Design review of the part built by this model. Coordinates are the model's own, in mm. A direction names the side the tool comes from. Coordinates: 2 decimals unless noted, no trailing zeros. Write each loop counter-clockwise with the first axis right and the second up, starting at its lowest first coordinate (ties: lowest second). Pieces come first, ordered by that corner, then holes.
Q1. The part is to be moulded in two halves that separate along X. For faces 1 (the face through (0, 4, 0)), 2 (the face through (-0.29, -2.23, 1.23)), 3 (the face through (2.64, -8.44, -0.99)), say which applies: +X half, -X half, draft (parallel to the pull), parting line (faces both ways), or undercut.
Q2. Add section B-B, the plane z = -1.6. Give the boundary of the cut face in (x, y) (3 decimals).
Q3. Add section D-D, the plane z = 1.5. Give the boundary of the cut face in (x, y), plus the area to 3 significant figures.
Q4. Add section C-C, the plane x = 4.25. Give the boundary of the cut face in (y, z), plus the area to 3 significant figures.
Q5. Clearance check with flat-ended pins moving along their axes: pin 1 Ø10 at (x, y) = (-2, 12) entering from +Z; pin 2 Ø2 at (x, z) = (-5, -1) entering from -Y; pin 3 Ø1 at (x, z) = (4.5, -1) entering from +Y. State where each tip first meets the part, or that it passes through.
Q6. Add section A-A, the plane y = 0. Give the boundary of the cut face in (x, z) (3 decimals).
Q7. To check wall thickness, follow probe 1 along X at (y, z) = (0, 1.75); probe 2 along Z at (x, y) = (-2, -6). State the ranges of each line that lie inside material, in increasing order.
Q8. Machinability: for faces 4 (the face through (-5, -2, -1)), 5 (the face through (0, 0, 0)), 6 (the face through (5, 2, -1)), 7 (the face through (5, -2, -1)), which of the approach directions +Z, -Z, +X, -X, +Y, -Y give a long, thin tool a straight path to every point of the face, cutting with its end or side? Answer none if there is none.
Autodesk Fusion 360 part; units mm, degrees
sketch "Sketch1" plane through (0, 0, 0) normal (0, 0, 1) x (1, 0, 0)
  circle A0 centre (0, 0) radius 3.5
  circle A1 centre (0, 0) radius 2.25
  circle A2 centre (0, 16.5) radius 2
  circle A3 centre (0, -14.5) radius 2
  circle A4 centre (-6.375, 0) radius 2
  circle A5 centre (6.375, 0) radius 2
  line L0 (0, 0) -> (0, 16.5) construction
  line L1 (-1.9917, 16.6818) -> (-3.4855, 0.3182)
  line L2 (-1.9893, -14.7069) -> (-3.4812, -0.3621)
  line L3 (1.9917, 16.6818) -> (3.4855, 0.3182)
  line L4 (1.9893, -14.7069) -> (3.4812, -0.3621)
  line L5 (-6.375, 2) -> (6.375, 2)
  line L6 (6.375, 2) -> (6.375, -2) construction
  line L7 (6.375, -2) -> (-6.375, -2)
  line L8 (-6.375, -2) -> (-6.375, 2) construction
  circle A6 centre (0, 0) radius 1.25
  circle A7 centre (0, 5) radius 0.625
  circle A8 centre (0, -5) radius 0.625
  point P0 (0, -16.5)
  point P1 (0, 18.5)
  point P2 (-8.375, 0)
  point P3 (8.375, 0)
  dimension "d1" = 7
  dimension "d2" = 4.5
  dimension "d5" = 35
  dimension "d7" = 4
  dimension "d8" = 16.75
  dimension "d9" = 14.5
  dimension "d12" = 2.5
  dimension "d14" = 5
  dimension "d15" = 1.25
  dimension "d22" = 5
extrude "Extrude1" add sketch "Sketch1" along normal blind 2.5 contours A0 A1 L5 L7 | A0 A1 L5 | A0 A1 L7 | A0 A1 L5 L7
extrude "Extrude2" add sketch "Sketch1" against normal blind 2 contours A0 A1 L5 L7 | A0 A5 L3 L4 L5 L7 | A0 L3 L5 | A0 L4 L7 | A0 A1 L5 | A0 A2 L1 L3 L5 | A0 A3 L2 L4 L7 | A0 A1 L7 | A0 A1 L5 L7 | A0 L1 L5 | A1 L5 | A1 L5 L7 | A2 | A5 | A0 L2 L7 | A1 L7 | A3 | A0 A4 L1 L2 L5 L7 | A4 | A6 | A7 | A8
extrude "Extrude4" cut sketch "Sketch1" along normal through all contours A7
pattern_linear "R-Pattern1" count 7 spacing 2 along (0, 1, 0) of "Extrude4"
extrude "Extrude5" cut sketch "Sketch1" along normal through all contours A8
pattern_linear "R-Pattern2" count 6 spacing 2 along (0, -1, 0) of "Extrude5"
extrude "Extrude6" cut sketch "Sketch1" along normal through all contours A6
Here are the results:
1. face 1: draft
1. face 2: undercut
1. face 3: +X half
2. outline: (-6.375, -2) - (-3.311, -2) - (-1.989, -14.707) arc R2 ccw to (1.989, -14.707) - (3.311, -2) - (6.375, -2) arc R2 ccw to (6.375, 2) - (3.332, 2) - (1.992, 16.682) arc R2 ccw to (-1.992, 16.682) - (-3.332, 2) - (-6.375, 2) arc R2 ccw to start
3. outline: circle Ø7 at (0, 0); hole circle Ø4.5 at (0, 0)
3. area: 22.6 mm2
4. outline: (-2, -2) - (2, -2) - (2, 0) - (-2, 0) - close
4. area: 8.00 mm2
5. pin 1: stops at z = 0
5. pin 2: stops at y = -2
5. pin 3: stops at y = 2
6. outline: (-8.375, -2) - (8.375, -2) - (8.375, 0) - (3.5, 0) - (3.5, 2.5) - (2.25, 2.5) - (2.25, 0) - (-2.25, 0) - (-2.25, 2.5) - (-3.5, 2.5) - (-3.5, 0) - (-8.375, 0) - close
7. probe 1: x = -3.5 to -2.25, 2.25 to 3.5
7. probe 2: z = -2 to 0
8. face 4: +Z, -Z, -X, -Y
8. face 5: +Z
8. face 6: +Z, -Z, +X, +Y
8. face 7: +Z, -Z, +X, -Y
